from build123d import *

# Parameters (mm, degrees)
F0_R        = 3.175
F0_W        = 6.35
F0_H        = 15.875
F1_DEPTH    = 3.175
F2_T1_DEPTH = 129.0963065702
F3_T1_DEPTH = 98.1970452562
F4_T1_DEPTH = 98.1970452562
F5_T1_DEPTH = 118.0977839421


# Not quite as in the source:
# - a fillet or chamfer that OpenCascade refuses, or shapes differently, is made with other operations: its cross-section is extruded or revolved along the edge and cut away or added
# - a length typed as a fraction of an inch, garbled in the dataset ("3 / 203.2 mm" for 3/8 in), is restored


with BuildPart() as f1:
    # F0 (on Front) → F1 (new body)
    with BuildSketch(Plane.XZ):
        Polygon((-0.2153298438, 38.1), (-51.0153298438, 38.1), (-51.0153298438, 0), (-51.0153298438, -8.2507394254), (-51.0153298438, -38.1), (50.5846701562, -38.1), (50.5846701562, 7.6242605746), (50.5846701562, 38.1), align=None)
        with Locations((-25.6096087396, -23.1753697127)):
            Circle(F0_R, mode=Mode.SUBTRACT)
        with Locations((-25.6145072252, -0.3132394254)):
            Rectangle(F0_W, F0_H, mode=Mode.SUBTRACT)
        with Locations((0, -23.1753697127)):
            Circle(F0_R, mode=Mode.SUBTRACT)
        with Locations((25.1914858818, -23.1753697127)):
            Circle(F0_R, mode=Mode.SUBTRACT)
        with Locations((-0.0039746718, -0.2589693381)):
            Rectangle(F0_W, F0_H, mode=Mode.SUBTRACT)
        with Locations((25.21736947, -0.2557926551)):
            Rectangle(F0_W, F0_H, mode=Mode.SUBTRACT)
        with Locations((-25.6096087396, 22.8621302873)):
            Circle(F0_R, mode=Mode.SUBTRACT)
        with Locations((0, 22.8621302873)):
            Circle(F0_R, mode=Mode.SUBTRACT)
        with Locations((25.1914858818, 22.8621302873)):
            Circle(F0_R, mode=Mode.SUBTRACT)
    extrude(amount=F1_DEPTH)

    # F2: fillet of radius 6.35 on 1 edges, made by hand

    # F2_s2 → F2_t1 (cut)
    with BuildSketch(Plane.YZ.offset(-64.7634831288)):
        with BuildLine():
            ThreePointArc((0, 38.1), (-2.324261314, 35.775738686), (-3.175, 32.600738686))
            Line((-3.175, 32.600738686), (-3.175, 38.1))
            Line((-3.175, 38.1), (0, 38.1))
        make_face()
    extrude(amount=F2_T1_DEPTH, mode=Mode.SUBTRACT)

    # F3: fillet of radius 6.35 on 1 edges, made by hand

    # F3_s2 → F3_t1 (cut)
    with BuildSketch(Plane.XY.offset(-51.8481532851)):
        with BuildLine():
            ThreePointArc((-51.0153298438, 0), (-48.6910685297, -2.324261314), (-45.5160685297, -3.175))
            Line((-45.5160685297, -3.175), (-51.0153298438, -3.175))
            Line((-51.0153298438, -3.175), (-51.0153298438, 0))
        make_face()
    extrude(amount=F3_T1_DEPTH, mode=Mode.SUBTRACT)

    # F4: fillet of radius 6.35 on 1 edges, made by hand

    # F4_s2 → F4_t1 (cut)
    with BuildSketch(Plane.XY.offset(-51.8481532851)):
        with BuildLine():
            ThreePointArc((50.5846701562, 0), (48.2604088422, -2.324261314), (45.0854088422, -3.175))
            Line((45.0854088422, -3.175), (50.5846701562, -3.175))
            Line((50.5846701562, -3.175), (50.5846701562, 0))
        make_face()
    extrude(amount=F4_T1_DEPTH, mode=Mode.SUBTRACT)

    # F5: fillet of radius 6.35 on 1 edges, made by hand

    # F5_s2 → F5_t1 (cut)
    with BuildSketch(Plane.YZ.offset(-59.2642218148)):
        with BuildLine():
            ThreePointArc((0, -38.1), (-2.324261314, -35.775738686), (-3.175, -32.600738686))
            Line((-3.175, -32.600738686), (-3.175, -38.1))
            Line((-3.175, -38.1), (0, -38.1))
        make_face()
    extrude(amount=F5_T1_DEPTH, mode=Mode.SUBTRACT)


solid = f1.part
Verification items for the finished model (mm, model axes). A direction names the side the tool comes from. Coordinates: 2 decimals unless noted, no trailing zeros. Order: outer loops, then holes, each group sorted by start corner. A loop starts at its lowest first (then second) coordinate and runs counter-clockwise, first axis right, second up. Notation, with made-up numbers: M -24.75,24 L 9.25,24 A20 ccw 9.25,31 Z; hole C -30,70 d1. An arc over 180 degrees is marked long. One line per item, written item: value. Start each with the question number.
Item 1: Sectioned sample at B-B on z = 25. Record the cut outline in (x, y) (3 decimals).
Item 2: Access from +Z, -Z, +X, -X, +Y, -Y to the whole of each face (thin tool, end or side, straight path). Record for faces 1 (the flat face through (-1, -3.175, 8)), 2 (the flat face through (0, -2, 7.679)).
Item 3: Depth check by flat-ended pin: P1, Ø1, axis at x = 24, y = -2, coming from the -Z side; P2, Ø1.6, axis at y = -1.5, z = -1.5, coming from the +X side; P3, Ø1.6, axis at y = -1.5, z = -2.5, coming from the -X side; P4, Ø5, axis at x = 0, z = 22.86, coming from the +Y side. Enter the tip coordinate at first touch or a pass-through.
Item 4: Sectioned sample at A-A on x = 0. Record the cut outline in (y, z) (3 decimals), then the cut area to 3 significant figures.
Item 5: Sectioned sample at D-D on z = -15.5. Record the cut outline in (x, y) (3 decimals).
Item 6: Thickness scan on probe 1 along Z at (x, y) = (0, -0.75); probe 2 along Z at (x, y) = (-26.5, -0.6); probe 3 along X at (y, z) = (-0.4, -5). Record the ranges inside material, lowest first.
Item 7: Sectioned sample at C-C on y = -1.7. Give the number of separate pieces and of enclosed holes in the cut face, then the cut area to 3 significant figures.
Item 8: Mould release check, pull along Z, two halves, no side actions. Record for faces 3 (the cylindrical face through (-0.93, -2.3, 35.82)), 4 (the cylindrical face through (-48.73, -2.3, -0.53)), 5 (the flat face through (22.042, -2, 0)): pulls with the +Z half, pulls with the -Z half, needs draft (parallel to the pull), parting line crosses it, or undercut.
Calculated:
1. outline: M -51.015,0 A6.35 ccw -45.516,-3.175 L -27.957,-3.175 L -27.957,0 Z; M -23.262,-3.175 L -2.347,-3.175 L -2.347,0 L -23.262,0 Z; M 2.347,-3.175 L 22.844,-3.175 L 22.844,0 L 2.347,0 Z; M 27.539,-3.175 L 45.085,-3.175 A6.35 ccw 50.585,0 L 27.539,0 Z
2. face 1: +Z, -Z, +X, -X, -Y
2. face 2: +Y, -Y
3. P1: z = -36.9
3. P2: x = 50.12
3. P3: x = -50.55
3. P4: through
4. outline: M -3.175,-32.601 A6.35 ccw 0,-38.1 L 0,-26.35 L -3.175,-26.35 Z; M -3.175,-20 L 0,-20 L 0,-8.196 L -3.175,-8.196 Z; M -3.175,7.679 L 0,7.679 L 0,19.687 L -3.175,19.687 Z; M -3.175,26.037 L 0,26.037 L 0,38.1 A6.35 ccw -3.175,32.601 Z
4. area: 141 mm^2
5. outline: M -51.015,0 A6.35 ccw -45.516,-3.175 L 45.085,-3.175 A6.35 ccw 50.585,0 Z
6. probe 1: -37.59 to -26.35, -20 to -8.2, 7.68 to 19.69, 26.04 to 37.59
6. probe 2: -37.71 to -26.22, -20.13 to -8.25, 7.62 to 19.81, 25.91 to 37.71
6. probe 3: -50.76 to -28.79, -22.44 to -3.18, 3.17 to 22.04, 28.39 to 50.33
7. separate pieces: 1
7. enclosed holes: 9
7. area: 6,750 mm^2
8. face 3: pulls with the +Z half
8. face 4: needs draft
8. face 5: undercut
